Geometry check sheet. Reference: drawing and pictorial views, mm from the part's lowest x, y, z. Give positions to 0.01 mm unless a question says otherwise; leave off trailing zeros. Write each loop counter-clockwise with the first axis right and the second up, starting at its lowest first coordinate (ties: lowest second). Pieces come first, ordered by that corner, then holes. Notation, with made-up numbers: (80, -23) -> (92, -23) arc R34 ccw to (92, 15) -> close; hole circle Ø7 at (41, 20.5). An arc over 180 degrees is marked (long way). Return JSON: item names as keys, results as strings.
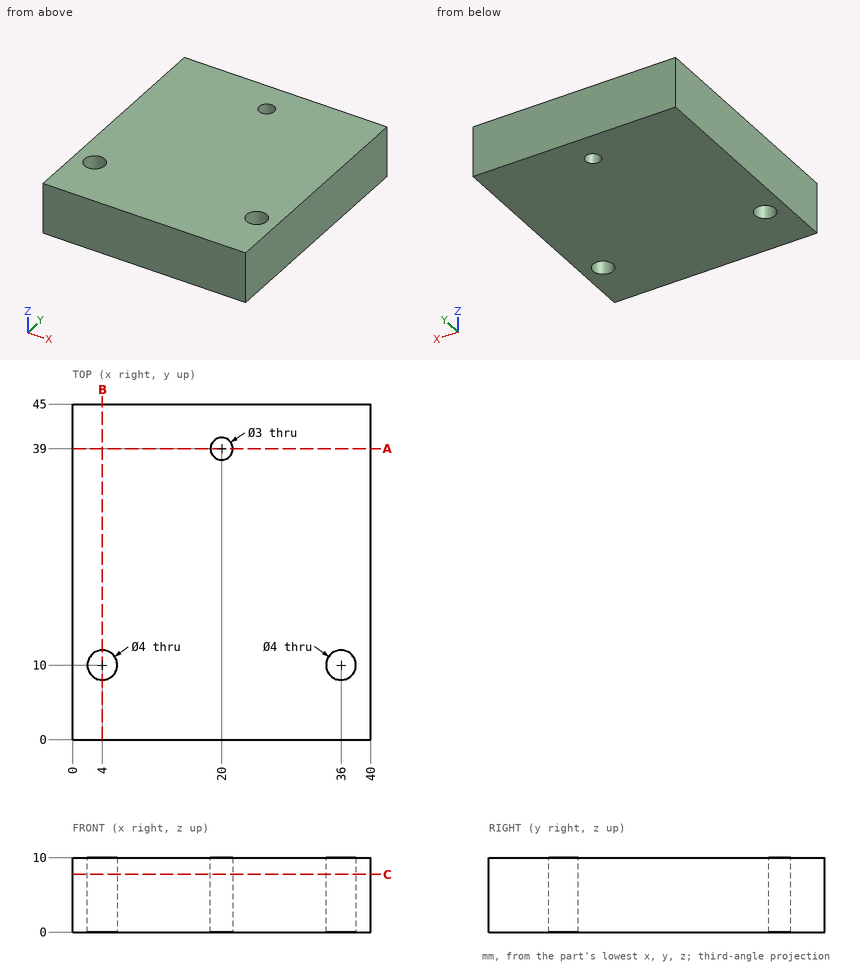
(1) Cross-section at B-B on x = 4. Enter the section's corners in (y, z), then the cut area to 3 significant figures.
Reply:
{"outline": "(0, 0) -> (8, 0) -> (8, 10) -> (0, 10) -> close; (12, 0) -> (45, 0) -> (45, 10) -> (12, 10) -> close", "area": "410 mm^2"}
(2) Thickness scan on L1, parallel to Y at x = 36, z = 6.25; L2, parallel to Y at x = 20, z = 2.75. Record the ranges inside material, lowest first.
Reply:
{"L1": "0 to 8, 12 to 45", "L2": "0 to 37.5, 40.5 to 45"}
(3) Cross-section at C-C on z = 7.75. Enter the section's corners in (x, y), then the cut area to 3 significant figures.
Reply:
{"outline": "(0, 0) -> (40, 0) -> (40, 45) -> (0, 45) -> close; hole circle Ø4 at (4, 10); hole circle Ø3 at (20, 39); hole circle Ø4 at (36, 10)", "area": "1,770 mm^2"}
(4) Cross-section at A-A on y = 39. Enter the section's corners in (x, z), then the cut area to 3 significant figures.
Reply:
{"outline": "(0, 0) -> (18.5, 0) -> (18.5, 10) -> (0, 10) -> close; (21.5, 0) -> (40, 0) -> (40, 10) -> (21.5, 10) -> close", "area": "370 mm^2"}
